Autodesk Inventor part; units mm, degrees
ref_plane "YZ Plane" through (0, 0, 0) normal (1, 0, 0) x (0, 1, 0)
ref_plane "XZ Plane" through (0, 0, 0) normal (0, 1, 0) x (-1, 0, 0)
ref_plane "XY Plane" through (0, 0, 0) normal (0, 0, 1) x (1, 0, 0)
sketch "Sketch1" plane through (0, 0, 0) normal (0, 1, 0) x (-1, 0, 0)
  line L0 (0, 0) -> (177.8, 0)
  line L1 (177.8, 0) -> (177.8, -190.5)
  line L2 (177.8, -190.5) -> (0, -190.5)
  line L3 (0, -190.5) -> (0, 0)
  line L4 (114.3, -3.175) -> (114.3, -187.325)
  line L5 (174.625, -93.6625) -> (3.175, -96.8375)
  line L6 (128.27, -69.85) -> (49.53, -69.85)
  line L7 (49.53, -69.85) -> (49.53, -120.65)
  line L8 (49.53, -120.65) -> (128.27, -120.65)
  line L9 (128.27, -120.65) -> (128.27, -69.85)
  line L10 (128.27, -69.85) -> (49.53, -120.65) construction
  line L11 (49.53, -69.85) -> (128.27, -120.65) construction
  line L12 (131.445, -66.675) -> (46.355, -66.675)
  line L13 (46.355, -66.675) -> (46.355, -123.825)
  line L14 (46.355, -123.825) -> (131.445, -123.825)
  line L15 (131.445, -123.825) -> (131.445, -66.675)
  line L16 (131.445, -66.675) -> (46.355, -123.825) construction
  line L17 (46.355, -66.675) -> (131.445, -123.825) construction
  line L18 (3.175, -187.325) -> (174.625, -187.325)
  line L19 (174.625, -187.325) -> (174.625, -3.175)
  line L20 (174.625, -3.175) -> (3.175, -3.175)
  line L21 (3.175, -3.175) -> (3.175, -187.325)
  line L22 (3.175, -187.325) -> (174.625, -3.175) construction
  line L23 (174.625, -187.325) -> (3.175, -3.175) construction
  line L24 (174.625, -93.6625) -> (174.625, -187.325)
  line L25 (174.625, -140.4938) -> (158.75, -140.4938)
  line L26 (174.625, -93.6625) -> (174.625, -3.175)
  line L27 (174.625, -48.4188) -> (209.55, -48.4188)
  line L28 (209.55, -48.4188) -> (171.45, -48.4188)
  line L29 (171.45, -48.4188) -> (171.45, -140.4938)
  line L30 (171.45, -140.4938) -> (158.75, -140.4938)
  point P0 (88.9, -95.25)
  point P1 (88.9, -95.25)
  dimension "d0" = 177.8
  dimension "d1" = 190.5
  dimension "d2" = 78.74
  dimension "d3" = 50.8
  dimension "d4" = 85.09
  dimension "d5" = 57.15
  dimension "d6" = 171.45
  dimension "d7" = 184.15
  dimension "d18" = 15.875
  dimension "d22" = 38.1
  dimension "d23" = 92.075
  dimension "d48" = 3.175
extrude "Extrusion1" add sketch "Sketch1" against normal blind 3.175 contours L19 L5 L29 L28 | L28 L29 L5 L15 L12 L4 L20 L19 | L0 L1 L2 L3 | L19 L25 L29 L5 | L29 L25 L19 L18 L4 L14 L15 L5 | L4 L12 L13 L5 L21 L20 | L15 L14 L4 L8 L9 L5 | L5 L9 L6 L4 L12 L15 | L4 L6 L7 L5 L13 L12 | L9 L8 L4 L5 | L5 L4 L6 L9 | L18 L21 L5 L13 L14 L4 | L4 L5 L7 L6 | L4 L8 L7 L5 | L14 L13 L5 L7 L8 L4
extrude "Extrusion2" add sketch "Sketch1" along normal blind 9.525 contours L15 L14 L4 L8 L9 L5 | L5 L9 L6 L4 L12 L15 | L4 L6 L7 L5 L13 L12 | L9 L8 L4 L5 | L5 L4 L6 L9 | L4 L5 L7 L6 | L4 L8 L7 L5 | L14 L13 L5 L7 L8 L4
extrude "Extrusion3" cut sketch "Sketch1" along normal blind 9.525 contours L9 L8 L4 L5 | L5 L4 L6 L9 | L4 L5 L7 L6 | L4 L8 L7 L5
extrude "Extrusion4" cut sketch "Sketch1" along normal blind 9.525 contours L9 L8 L4 L5 | L5 L4 L6 L9 | L4 L5 L7 L6 | L4 L8 L7 L5
extrude "Extrusion5" add sketch "Sketch1" along normal blind 22.225
sketch "Sketch2" plane through (0, -3.175, -190.5) normal (0, 0, -1) x (-1, 0, 0)
  line L0 (177.8, 25.4) -> (177.8, 0)
  line L1 (177.8, 25.4) -> (123.825, 25.4)
  line L2 (123.825, 25.4) -> (123.825, 0)
  line L3 (0, 0) -> (177.8, 0)
  line L4 (177.8, 0) -> (177.8, 15.875)
  line L5 (177.8, 15.875) -> (123.825, 15.875)
  line L6 (177.8, 15.875) -> (153.9875, 15.875)
  line L7 (153.9875, 15.875) -> (141.2875, 15.875)
  line L8 (150.8125, 12.7) -> (157.1625, 12.7)
  line L9 (157.1625, 12.7) -> (157.1625, 19.05)
  line L10 (157.1625, 19.05) -> (150.8125, 19.05)
  line L11 (150.8125, 19.05) -> (150.8125, 12.7)
  line L12 (150.8125, 12.7) -> (157.1625, 19.05) construction
  line L13 (157.1625, 12.7) -> (150.8125, 19.05) construction
  line L14 (144.4625, 12.7) -> (138.1125, 12.7)
  line L15 (138.1125, 12.7) -> (138.1125, 19.05)
  line L16 (138.1125, 19.05) -> (144.4625, 19.05)
  line L17 (144.4625, 19.05) -> (144.4625, 12.7)
  line L18 (144.4625, 12.7) -> (138.1125, 19.05) construction
  line L19 (138.1125, 12.7) -> (144.4625, 19.05) construction
  line L20 (141.2875, 15.875) -> (127, 15.875)
  line L21 (127, 15.875) -> (25.4, 15.875)
  line L22 (141.2875, 15.875) -> (128.5875, 15.875)
  line L23 (125.4125, 12.7) -> (131.7625, 12.7)
  line L24 (131.7625, 12.7) -> (131.7625, 19.05)
  line L25 (131.7625, 19.05) -> (125.4125, 19.05)
  line L26 (125.4125, 19.05) -> (125.4125, 12.7)
  line L27 (125.4125, 12.7) -> (131.7625, 19.05) construction
  line L28 (131.7625, 12.7) -> (125.4125, 19.05) construction
  line L29 (22.225, 19.05) -> (28.575, 19.05)
  line L30 (28.575, 19.05) -> (28.575, 12.7)
  line L31 (28.575, 12.7) -> (22.225, 12.7)
  line L32 (22.225, 12.7) -> (22.225, 19.05)
  line L33 (22.225, 19.05) -> (28.575, 12.7) construction
  line L34 (28.575, 19.05) -> (22.225, 12.7) construction
  line L35 (0, 0) -> (0, 25.4)
  point P0 (0, 3.175)
  dimension "d25" = 15.875
  dimension "d27" = 12.7
  dimension "d28" = 6.35
  dimension "d29" = 6.35
  dimension "d30" = 6.35
  dimension "d31" = 6.35
  dimension "d32" = 14.2875
  dimension "d36" = 101.6
  dimension "d38" = 12.7
  dimension "d39" = 6.35
  dimension "d40" = 6.35
  dimension "d41" = 6.35
  dimension "d42" = 6.35
  dimension "d44" = 25.4
  dimension "d45" = 53.975
extrude "Extrusion6" cut sketch "Sketch2" against normal blind 190.5 contours L30 L31 L32 L29 | L9 L8 L11 L5 | L5 L11 L10 L9 | L26 L25 L24 L5 | L5 L24 L23 L26 | L17 L14 L15 L5 | L5 L15 L16 L17
properties part number "RCcar_full build"
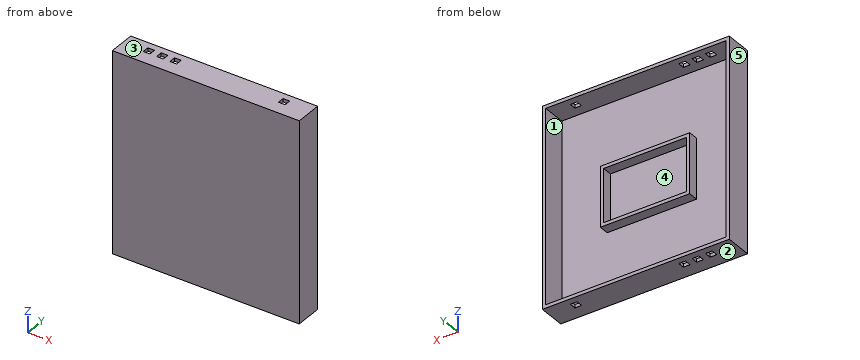
The model under review builds one solid part; all positions refer to its coordinate system, in mm. Face numbers are marked on the shaded views. A direction names the side the tool comes from. Coordinates: 2 decimals unless noted, no trailing zeros. Order: outer loops, then holes, each group sorted by start corner. A loop starts at its lowest first (then second) coordinate and runs counter-clockwise, first axis right, second up. Notation, with made-up numbers: M 23.25,73.5 L 62.25,73.5 A24 ccw 62.25,105.5 Z; hole C -4.5,57.25 d8. An arc over 180 degrees is marked long. One line per question, with ' | ' between items.
(1) The part is to be moulded in two halves that separate along X. For the marked faces 3, 4 and 5, say which applies: +X half, -X half, draft (parallel to the pull), parting line (faces both ways), or undercut.
Geometry results:
face 3: draft | face 4: undercut | face 5: -X half
(2) Add section B-B, the plane x = -155. Write out the cut boundary in (y, z) (3 decimals), then the cut area to 3 significant figures.
Geometry results:
outline: M -3.175,-190.5 L 9.525,-190.5 L 9.525,-187.325 L 0,-187.325 L 0,-3.175 L 9.525,-3.175 L 9.525,0 L -3.175,0 Z; M 15.875,-190.5 L 22.225,-190.5 L 22.225,-187.325 L 15.875,-187.325 Z; M 15.875,-3.175 L 22.225,-3.175 L 22.225,0 L 15.875,0 Z | area: 706 mm²
(3) Add section D-D, the plane z = -150.5. Write out the cut boundary in (x, y) (3 decimals), then the cut area to 3 significant figures.
Geometry results:
outline: M -177.8,-3.175 L 0,-3.175 L 0,22.225 L -3.175,22.225 L -3.175,0 L -174.625,0 L -174.625,22.225 L -177.8,22.225 Z | area: 706 mm²
(4) Insertion check: pin 1 (15 mm diameter, centred on x = -95, z = -106.5, fed in from +Y); pin 2 (2 mm diameter, centred on x = -25, y = 11, fed in from +Z). Each pin has a flat end and moves straight along its axis. Give the tip position at first contact, or say it passes through.
Geometry results:
pin 1: stops at y = 0 | pin 2: passes through
(5) For probe 1 along Z at (x, y) = (-49, 8.5) (3 decimals); probe 2 along Z at (x, y) = (-32, 0.75) (3 decimals); probe 3 along X at (y, z) = (7.75, -37) (3 decimals), list the stretches that pass through material, from the lowest coordinate up. Write a range as from..to.
Geometry results:
probe 1: z = -190.5..-187.325, -123.825..-66.675, -3.175..0 | probe 2: z = -190.5..-187.325, -3.175..0 | probe 3: x = -177.8..-174.625, -3.175..0
(6) Add section C-C, the plane y = 18.5. Write out the cut boundary in (x, z) (3 decimals), then the cut area to 3 significant figures.
Geometry results:
outline: M -177.8,-190.5 L 0,-190.5 L 0,0 L -177.8,0 Z; hole M -174.625,-187.325 L -3.175,-187.325 L -3.175,-3.175 L -174.625,-3.175 Z | area: 2,300 mm²
(7) Machinability: for the marked faces 1 and 2, which of the approach directions +Z, -Z, +X, -X, +Y, -Y give a long, thin tool a straight path to every point of the face, cutting with its end or side? Answer none if there is none.
Geometry results:
face 1: +Y | face 2: -Z, +X, -X, +Y, -Y
(8) Add section A-A, the plane y = 4. Write out the cut boundary in (x, z) (3 decimals), then the cut area to 3 significant figures.
Geometry results:
outline: M -177.8,-190.5 L 0,-190.5 L 0,0 L -177.8,0 Z; M -131.445,-123.825 L -46.355,-123.825 L -46.355,-66.675 L -131.445,-66.675 Z; hole M -174.625,-187.325 L -3.175,-187.325 L -3.175,-3.175 L -174.625,-3.175 Z; hole M -128.27,-120.65 L -49.53,-120.65 L -49.53,-69.85 L -128.27,-69.85 Z | area: 3,160 mm²
